Can you work these out from the drawing? Everything is in mm from the part's minimum corner. A direction names the side the tool comes from. Round coordinates to 2 decimals unless told otherwise and drop trailing zeros. Order: outer loops, then holes, each group sorted by start corner. A loop starts at its lowest first (then second) coordinate and runs counter-clockwise, first axis right, second up. Notation, with made-up numbers: (3.25, 47.25) -> (56.25, 47.25) arc R23 cw to (56.25, 68.25) -> close; hole circle Ø3 at (-16, -10.75). An arc over 180 degrees is marked (long way). One line per item, written item: value.
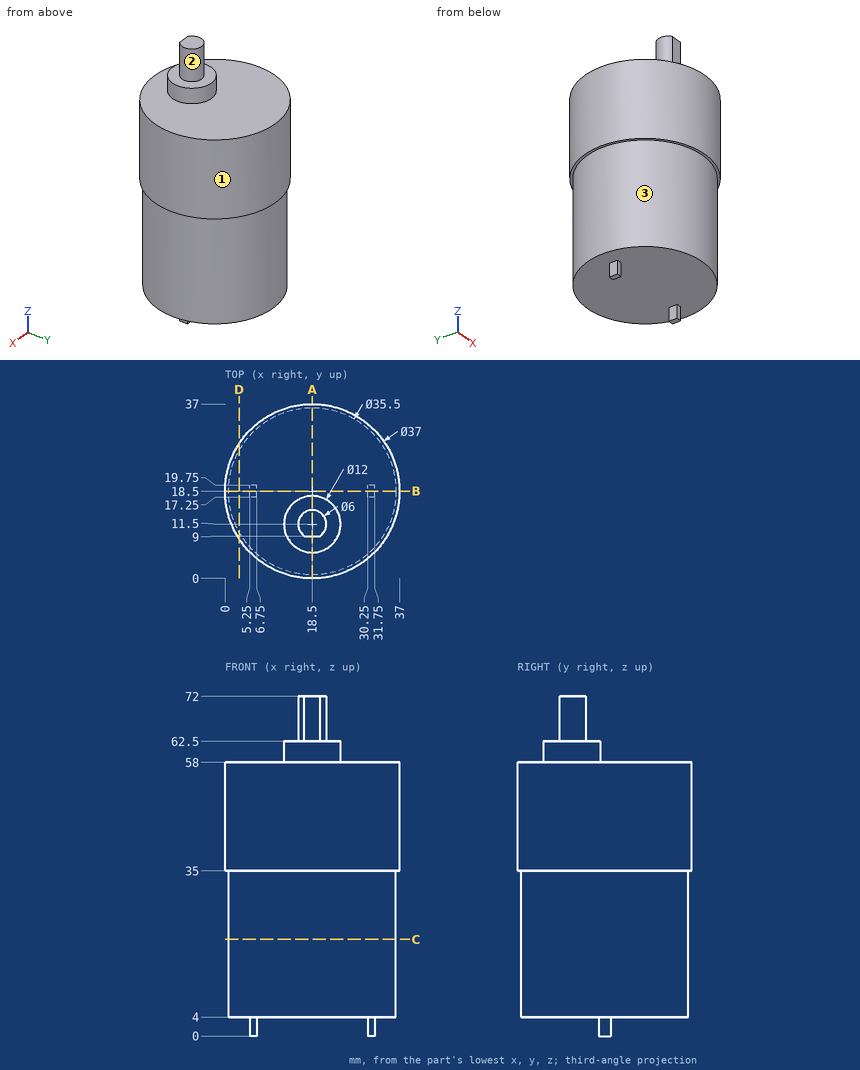
Q1. I want a section at B-B on y = 18.5. Write out the boundary of the cut face in (x, z), then the cut area to 3 significant figures.
Answers:
outline: (0, 35) -> (0.75, 35) -> (0.75, 4) -> (5.25, 4) -> (5.25, 0) -> (6.75, 0) -> (6.75, 4) -> (30.25, 4) -> (30.25, 0) -> (31.75, 0) -> (31.75, 4) -> (36.25, 4) -> (36.25, 35) -> (37, 35) -> (37, 58) -> (0, 58) -> close
area: 1,960 mm2
Q2. I want a section at C-C on z = 20.5. Write out the boundary of the cut face in (x, y).
Answers:
outline: circle Ø35.5 at (18.5, 18.5)
Q3. I want a section at D-D on x = 3. Write out the boundary of the cut face in (y, z), then the cut area to 3 significant figures.
Answers:
outline: (8.4, 35) -> (9.85, 35) -> (9.85, 4) -> (27.15, 4) -> (27.15, 35) -> (28.6, 35) -> (28.6, 58) -> (8.4, 58) -> close
area: 1,000 mm2
Q4. For P1, Ø3, axis at x = 10.5, z = 49.5, coming from the +Y side; P2, Ø18.5, axis at x = 16.5, y = 18, coming from the -Z side; P3, Ø10, axis at x = 8, y = 19.5, coming from the +Z side, each with a flat end and sliding along its axis, tell me the tip position at first contact or that it passes through.
Answers:
P1: y = 35.82
P2: z = 4
P3: z = 58
Q5. I need wall thicknesses on line 1 along Z through (x, y) = (11, 7.5); line 2 along Z through (x, y) = (8, 33.5); line 3 along X through (y, z) = (5, 28). Which ranges of each line are inside material? Lowest first, please.
Answers:
line 1: 4 to 58
line 2: 35 to 58
line 3: 6.98 to 30.02
Q6. I want a section at A-A on x = 18.5. Write out the boundary of the cut face in (y, z), then the cut area to 3 significant figures.
Answers:
outline: (0, 35) -> (0.75, 35) -> (0.75, 4) -> (36.25, 4) -> (36.25, 35) -> (37, 35) -> (37, 58) -> (17.5, 58) -> (17.5, 62.5) -> (14.5, 62.5) -> (14.5, 72) -> (9, 72) -> (9, 62.5) -> (5.5, 62.5) -> (5.5, 58) -> (0, 58) -> close
area: 2,060 mm2
Q7. Which directions (+Z, -Z, +X, -X, +Y, -Y) give clear straight access to the entire face, cutting with the end or side of a thin tool? Please do the marked faces 1, 2 and 3.
Answers:
face 1: +Z, -Z
face 2: +Z
face 3: -Z
